Geometry: final body of the model. Coordinates: model frame, mm. A direction names the side the tool comes from. Round coordinates to 2 decimals unless told otherwise and drop trailing zeros. Write each loop counter-clockwise with the first axis right and the second up, starting at its lowest first coordinate (ties: lowest second). Pieces come first, ordered by that corner, then holes. Notation, with made-up numbers: M -19.5,12 L -3.5,12 A23 cw -3.5,27 Z; hole C -1.75,25.25 d9. An arc over 180 degrees is marked long. Put each result on its own line as item: value. Start each with the question number.
Autodesk Inventor part; units mm, degrees
ref_plane "to_screw1_XY" through (12, 3.5355, 3.5355) normal (0, 0.7071, 0.7071) x (1, 0, 0)
ref_plane "to_screw1_YZ" through (12, 3.5355, 3.5355) normal (1, 0, 0) x (0, 0.7071, -0.7071)
ref_plane "to_screw1_ZX" through (12, 3.5355, 3.5355) normal (0, 0.7071, -0.7071) x (0, 0.7071, 0.7071)
sketch "Sketch_1" plane through (0, 0, 0) normal (0, 0, 1) x (1, 0, 0)
  line L0 (20, 0) -> (0, 0)
  line L1 (0, 15) -> (0, 5)
  line L2 (0, 5) -> (20, 5)
  line L3 (20, 5) -> (20, 7)
  line L4 (20, 7) -> (5, 7)
  line L5 (5, 7) -> (5, 15)
  line L6 (5, 15) -> (0, 15)
revolve "Revolution1" add sketch "Sketch_1" angle 360 about axis through (20, 0, 0) along (1, 0, 0)
sketch "Sketch_3" plane through (0, 0, 0) normal (0, -0.7071, 0.7071) x (1, 0, 0)
  line L0 (12, 4.5) -> (12, 7)
  line L1 (12, 7) -> (14, 7)
  line L2 (14, 7) -> (13.621, 6.621)
  line L3 (13.621, 6.621) -> (13.621, 4.5)
  line L4 (13.621, 4.5) -> (12, 4.5)
  line L5 (12, 4.5) -> (12, 7)
revolve "Revolution2" cut sketch "Sketch_3" angle 360 about axis through (12, 3.182, 3.182) along (0, -0.7071, -0.7071)
thread "Thread1"
sketch "Sketch3" plane through (5, 0, 0) normal (1, 0, 0) x (0, 0, -1)
  point P0 (0, 11)
hole "Hole1" at (5, 11, 0) direction (-1, 0, 0) diameter 4.5 depth 5
sketch "Sketch4" plane through (5, 0, 0) normal (1, 0, 0) x (0, 0, -1)
  point P0 (0, -11)
hole "Hole2" at (5, -11, 0) direction (-1, 0, 0) diameter 4.5 depth 5
sketch "Sketch5" plane through (5, 0, 0) normal (1, 0, 0) x (0, 0, -1)
  point P0 (-11, 0)
hole "Hole3" at (5, 0, 11) direction (-1, 0, 0) diameter 4.5 depth 5
sketch "Sketch6" plane through (5, 0, 0) normal (1, 0, 0) x (0, 0, -1)
  point P0 (11, 0)
hole "Hole4" at (5, 0, -11) direction (-1, 0, 0) diameter 4.5 depth 5
sketch "Sketch_2" plane through (0, 0, 0) normal (0, -0.7071, -0.7071) x (1, 0, 0)
  line L0 (12, 4.5) -> (12, 7)
  line L1 (12, 7) -> (14, 7)
  line L2 (14, 7) -> (13.621, 6.621)
  line L3 (13.621, 6.621) -> (13.621, 4.5)
  line L4 (13.621, 4.5) -> (12, 4.5)
  line L5 (12, 4.5) -> (12, 7)
revolve "Revolution3" cut sketch "Sketch_2" angle 360 about axis through (12, -3.182, 3.182) along (0, 0.7071, -0.7071)
thread "Thread2"
ref_plane "to_screw1_XY" through (12, 3.5355, 3.5355) normal (0, 0.7071, 0.7071) x (1, 0, 0)
ref_plane "to_screw1_YZ" through (12, 3.5355, 3.5355) normal (1, 0, 0) x (0, 0.7071, -0.7071)
ref_plane "to_screw1_ZX" through (12, 3.5355, 3.5355) normal (0, 0.7071, -0.7071) x (0, 0.7071, 0.7071)
ref_plane "to_screw2_XY" through (12, -3.5355, 3.5355) normal (0, -0.7071, 0.7071) x (1, 0, 0)
ref_plane "to_screw2_YZ" through (12, -3.5355, 3.5355) normal (1, 0, 0) x (0, 0.7071, 0.7071)
ref_plane "to_screw2_ZX" through (12, -3.5355, 3.5355) normal (0, 0.7071, 0.7071) x (0, -0.7071, 0.7071)
properties part number "STHRB10M-MB_b" material "ステンレス鋼"
1) Section D-D, the plane z = -3. Output: boundary loops of the cut face in (x, y).
2) Section A-A, the plane z = 0. Output: boundary loops of the cut face in (x, y), and give its area (3 significant figures).
3) Access query for faces 5 (the face through (2.46, 8.77, 0.29)), 6 (the face through (5, 6.5, -3.1)). Directions: +Z, -Z, +X, -X, +Y, -Y. A direction counts if a zero-diameter tool reaches every point of the face in a straight line with its end or side. Return the directions, or none.
4) Ray query, probe 1 along Z at (x, y) = (1.75, 0); probe 2 along Z at (x, y) = (12, 0); probe 3 along X at (y, z) = (-7.75, 3.25). Return the intervals inside material, ascending.
5) First-contact query: pin 1 (2 mm diameter, centred on x = 3.5, z = 10.5, fed in from +Y); pin 2 (3 mm diameter, centred on x = 14, z = 2.5, fed in from -Y); pin 3 (6 mm diameter, centred on y = 0, z = -11, fed in from +X). Flat tips, straight axial feed; report the tip coordinate or a pass-through.
6) Section C-C, the plane x = 2.75. Output: boundary loops of the cut face in (y, z), and give its area (3 significant figures).
7) Draft query along X for faces 1 (the face through (0, -4, 4)), 2 (the face through (2.465, -0.099, 13.248)), 3 (the face through (13.497, -3.565, 4.443)), 4 (the face through (13.497, 4.443, 3.565)). Return one class per face: +X half, -X half, draft (parallel to the pull), parting line (faces both ways), or undercut.
Solved:
1. outline: M 0,-14.7 L 5,-14.7 L 5,-6.32 L 20,-6.32 L 20,-4 L 0,-4 Z; M 0,4 L 20,4 L 20,6.32 L 5,6.32 L 5,14.7 L 0,14.7 Z
2. outline: M 0,-15 L 5,-15 L 5,-13.25 L 0,-13.25 Z; M 0,-8.75 L 5,-8.75 L 5,-7 L 20,-7 L 20,-5 L 0,-5 Z; M 0,5 L 20,5 L 20,7 L 5,7 L 5,8.75 L 0,8.75 Z; M 0,13.25 L 5,13.25 L 5,15 L 0,15 Z
2. area: 115 mm2
3. face 5: +X, -X
3. face 6: +X
4. probe 1: z = -15 to -13.25, -8.75 to -5, 5 to 8.75, 13.25 to 15
4. probe 2: z = -7 to -5, 5 to 7
4. probe 3: x = 0 to 5
5. pin 1: stops at y = 11.61
5. pin 2: stops at y = -6.93
5. pin 3: stops at x = 5
6. outline: C 0,0 d30; hole C -11,0 d4.5; hole C 0,0 d10; hole C 0,-11 d4.5; hole C 0,11 d4.5; hole C 11,0 d4.5
6. area: 565 mm2
7. face 1: -X half
7. face 2: draft
7. face 3: undercut
7. face 4: undercut
